Autodesk Inventor part; units mm, degrees
ref_plane "YZ Plane" through (0, 0, 0) normal (1, 0, 0) x (0, 1, 0)
ref_plane "XZ Plane" through (0, 0, 0) normal (0, 1, 0) x (-1, 0, 0)
ref_plane "XY Plane" through (0, 0, 0) normal (0, 0, 1) x (1, 0, 0)
sketch "スケッチ1" plane through (0, 0, 0) normal (0, 1, 0) x (-1, 0, 0)
  line L0 (-3, 0.3) -> (-3, 3.7)
  line L1 (-3.3, 4) -> (-3.7, 4)
  line L2 (-4, 3) -> (-4, 1)
  line L3 (-4, 1) -> (-6, 1)
  line L4 (-6, 1) -> (-6, 0)
  line L5 (-6, 0) -> (-3.3, 0)
  line L6 (-3, 3.7) -> (-3.3, 4)
  line L7 (-3, 0.3) -> (-3.3, 0)
  line L8 (-3.7, 4) -> (-4, 3)
  line L9 (0, -0.8) -> (0, 4.8)
  point P0 (0, 0)
  point P1 (-3, 0)
  point P2 (-3, 4)
  point P3 (-4, 4)
  dimension "d2" = 1
  dimension "d9" = 1
  dimension "d11" = 6
  dimension "d12" = 8
  dimension "d13" = 12
  dimension "d14" = 0.3
  dimension "d15" = 0.3
  dimension "d16" = 0.3
  dimension "d17" = 0.3
  dimension "d18" = 0.3
  dimension "d19" = 4
revolve "回転1" add sketch "スケッチ1" angle 360 about axis through (0, 0, -10) along (0, 0, 1)
sketch "스케치2" plane through (0, 0, 0) normal (0, 0, -1) x (-1, 0, 0)
  circle A0 centre (0, 0) radius 3.3
  circle A1 centre (0, 0) radius 6
  circle A2 centre (0, 0) radius 3.025
  dimension "d20" = 6.05
extrude "돌출1" cut sketch "스케치2" against normal up to surface (4 mm away) contours A2
equation "\"d15\" = d14"
equation "\"d16\" = d14"
equation "\"d17\" = d16"
equation "\"d18\" = d14"
properties part number "80F-0603"
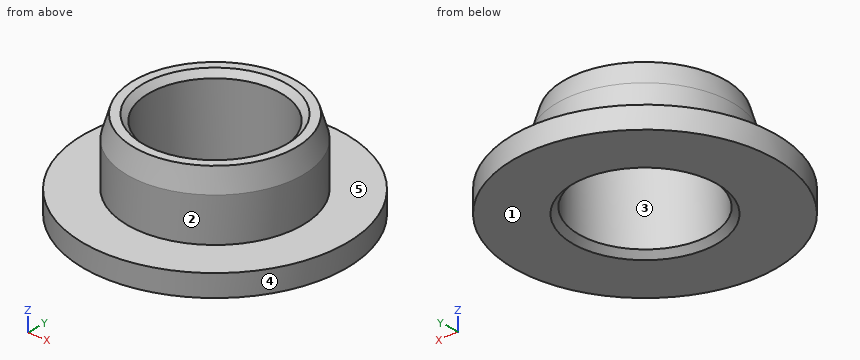
Check sheet for the modelled part. Datum: model origin and axes. Units: mm. Face numbers are marked on the shaded views. A direction names the side the tool comes from. Give positions to 0.01 mm unless a question says otherwise; leave off trailing zeros. Loops run counter-clockwise (first coordinate to the right, second up) from the corner with the lowest first, then second, coordinate; pieces in that order, holes last. Notation, with made-up numbers: M 0.5,0.5 L 40.5,0.5 A24 cw 40.5,34.5 Z; hole C 36,23.25 d11. An arc over 180 degrees is marked long. Answer in a Markdown table with one row per item.
1) Thickness scan on line 1 (Y direction, x = 0, z = 2.5) (3 decimals); line 2 (Z direction, x = 2.25, y = -5); line 3 (X direction, y = -2, z = 0.4). Record the ranges inside material, lowest first.
Solutions:
| item | result |
|---|---|
| line 1 | y = -4 to -3.025, 3.025 to 4 |
| line 2 | z = 0 to 1 |
| line 3 | x = -5.66 to -2.27, 2.27 to 5.66 |
2) Tool access check on the marked faces 4 and 5. Record the directions out of +Z, -Z, +X, -X, +Y, -Y that give a thin tool (end or side, any length) a straight path to the whole face; none if there is none.
Solutions:
| item | result |
|---|---|
| face 4 | +Z, -Z |
| face 5 | +Z |
3) Cross-section at C-C (z = 1.65). Enter the section's corners in (x, y) (3 decimals), plus the area to 3 significant figures.
Solutions:
| item | result |
|---|---|
| outline | C 0,0 d8; hole C 0,0 d6.05 |
| area | 21.5 mm^2 |
4) Mould release check, pull along X, two halves, no side actions. Record for the marked faces 1, 2 and 3: released by +X, released by -X, zero draft, split by the parting line, or undercut.
Solutions:
| item | result |
|---|---|
| face 1 | zero draft |
| face 2 | split by the parting line |
| face 3 | undercut |
5) Depth check by flat-ended pin: pin 1 (1 mm diameter, centred on x = -4, y = -4, fed in from +Z). Enter the tip coordinate at first touch or a pass-through.
Solutions:
| item | result |
|---|---|
| pin 1 | stops at z = 1 |
6) Cross-section at A-A (y = 0). Enter the section's corners in (x, z) (3 decimals).
Solutions:
| item | result |
|---|---|
| outline | M -6,0 L -3.3,0 L -3.025,0.275 L -3.025,3.725 L -3.3,4 L -3.7,4 L -4,3 L -4,1 L -6,1 Z; M 3.025,0.275 L 3.3,0 L 6,0 L 6,1 L 4,1 L 4,3 L 3.7,4 L 3.3,4 L 3.025,3.725 Z |
